Autodesk Inventor part; units mm, degrees
ref_plane "YZ Plane" through (0, 0, 0) normal (1, 0, 0) x (0, 1, 0)
ref_plane "XZ Plane" through (0, 0, 0) normal (0, 1, 0) x (-1, 0, 0)
ref_plane "XY Plane" through (0, 0, 0) normal (0, 0, 1) x (1, 0, 0)
sketch "Sketch1" plane through (0, 0, 0) normal (0, 0, 1) x (1, 0, 0)
  circle A0 centre (0, 0) radius 17.5
  dimension "d0" = 35
extrude "Extrusion1" add sketch "Sketch1" along normal blind 6
sketch "Sketch7" plane through (0, 0, 6) normal (0, 0, 1) x (1, 0, 0)
  circle A0 centre (0, 0) radius 17.5 construction
  line L0 (0, 0) -> (15, 0) construction
  circle A1 centre (0, 0) radius 17.5
  arc A2 (21.3853, 0.9) -> (17.3853, 2) centre (15.4462, -12.8741) ccw
  arc A3 (21.3853, -0.9) -> (21.3853, 0.9) centre (1.4056, 0) ccw
  arc A4 (17.3853, -2) -> (21.3853, -0.9) centre (15.4462, 12.8741) ccw
  arc A5 (17.3853, -2) -> (17.3853, 2) centre (0, 0) ccw
  arc A6 (20.2655, 6.8885) -> (16.1176, 6.817) centre (18.4476, -8.0009) ccw
  arc A7 (17.2446, 2.979) -> (16.1176, 6.817) centre (0, 0) ccw
  arc A8 (17.2446, 2.979) -> (20.7726, 5.1614) centre (11.1935, 16.7043) ccw
  arc A9 (20.7726, 5.1614) -> (20.2655, 6.8885) centre (1.3487, 0.396) ccw
  arc A10 (17.5039, 12.3189) -> (13.5442, 11.0817) centre (19.9545, -2.4796) ccw
  arc A11 (15.7068, 7.7167) -> (13.5442, 11.0817) centre (0, 0) ccw
  arc A12 (15.7068, 7.7167) -> (18.4771, 10.8047) centre (6.0339, 19.1813) ccw
  arc A13 (18.4771, 10.8047) -> (17.5039, 12.3189) centre (1.1825, 0.7599) ccw
  arc A14 (13.3242, 16.7513) -> (9.8735, 14.4487) centre (19.8447, 3.2427) ccw
  arc A15 (12.8965, 11.8292) -> (9.8735, 14.4487) centre (0, 0) ccw
  arc A16 (12.8965, 11.8292) -> (14.6846, 15.5726) centre (0.3855, 20.1042) ccw
  arc A17 (14.6846, 15.5726) -> (13.3242, 16.7513) centre (0.9205, 1.0623) ccw
  arc A18 (8.0651, 19.8267) -> (5.4029, 16.6451) centre (18.1273, 8.7023) ccw
  arc A19 (9.0414, 14.9834) -> (5.4029, 16.6451) centre (0, 0) ccw
  arc A20 (9.0414, 14.9834) -> (9.7025, 19.0789) centre (-5.2941, 19.3985) ccw
  arc A21 (9.7025, 19.0789) -> (8.0651, 19.8267) centre (0.5839, 1.2786) ccw
  arc A22 (2.1526, 21.2958) -> (0.4945, 17.493) centre (14.9413, 13.4568) ccw
  arc A23 (4.4538, 16.9238) -> (0.4945, 17.493) centre (0, 0) ccw
  arc A24 (4.4538, 16.9238) -> (3.9343, 21.0396) centre (-10.5449, 17.1212) ccw
  arc A25 (3.9343, 21.0396) -> (2.1526, 21.2958) centre (0.2, 1.3913) ccw
  arc A26 (-3.9343, 21.0396) -> (-4.4538, 16.9238) centre (10.5449, 17.1212) ccw
  arc A27 (-0.4945, 17.493) -> (-4.4538, 16.9238) centre (0, 0) ccw
  arc A28 (-0.4945, 17.493) -> (-2.1526, 21.2958) centre (-14.9413, 13.4568) ccw
  arc A29 (-2.1526, 21.2958) -> (-3.9343, 21.0396) centre (-0.2, 1.3913) ccw
  arc A30 (-9.7025, 19.0789) -> (-9.0414, 14.9834) centre (5.2941, 19.3985) ccw
  arc A31 (-5.4029, 16.6451) -> (-9.0414, 14.9834) centre (0, 0) ccw
  arc A32 (-5.4029, 16.6451) -> (-8.0651, 19.8267) centre (-18.1273, 8.7023) ccw
  arc A33 (-8.0651, 19.8267) -> (-9.7025, 19.0789) centre (-0.5839, 1.2786) ccw
  arc A34 (-14.6846, 15.5726) -> (-12.8965, 11.8292) centre (-0.3855, 20.1042) ccw
  arc A35 (-9.8735, 14.4487) -> (-12.8965, 11.8292) centre (0, 0) ccw
  arc A36 (-9.8735, 14.4487) -> (-13.3242, 16.7513) centre (-19.8447, 3.2427) ccw
  arc A37 (-13.3242, 16.7513) -> (-14.6846, 15.5726) centre (-0.9205, 1.0623) ccw
  arc A38 (-18.4771, 10.8047) -> (-15.7068, 7.7167) centre (-6.0339, 19.1813) ccw
  arc A39 (-13.5442, 11.0817) -> (-15.7068, 7.7167) centre (0, 0) ccw
  arc A40 (-13.5442, 11.0817) -> (-17.5039, 12.3189) centre (-19.9545, -2.4796) ccw
  arc A41 (-17.5039, 12.3189) -> (-18.4771, 10.8047) centre (-1.1825, 0.7599) ccw
  arc A42 (-20.7726, 5.1614) -> (-17.2446, 2.979) centre (-11.1935, 16.7043) ccw
  arc A43 (-16.1176, 6.817) -> (-17.2446, 2.979) centre (0, 0) ccw
  arc A44 (-16.1176, 6.817) -> (-20.2655, 6.8885) centre (-18.4476, -8.0009) ccw
  arc A45 (-20.2655, 6.8885) -> (-20.7726, 5.1614) centre (-1.3487, 0.396) ccw
  arc A46 (-21.3853, -0.9) -> (-17.3853, -2) centre (-15.4462, 12.8741) ccw
  arc A47 (-17.3853, 2) -> (-17.3853, -2) centre (0, 0) ccw
  arc A48 (-17.3853, 2) -> (-21.3853, 0.9) centre (-15.4462, -12.8741) ccw
  arc A49 (-21.3853, 0.9) -> (-21.3853, -0.9) centre (-1.4056, 0) ccw
  arc A50 (-20.2655, -6.8885) -> (-16.1176, -6.817) centre (-18.4476, 8.0009) ccw
  arc A51 (-17.2446, -2.979) -> (-16.1176, -6.817) centre (0, 0) ccw
  arc A52 (-17.2446, -2.979) -> (-20.7726, -5.1614) centre (-11.1935, -16.7043) ccw
  arc A53 (-20.7726, -5.1614) -> (-20.2655, -6.8885) centre (-1.3487, -0.396) ccw
  arc A54 (-17.5039, -12.3189) -> (-13.5442, -11.0817) centre (-19.9545, 2.4796) ccw
  arc A55 (-15.7068, -7.7167) -> (-13.5442, -11.0817) centre (0, 0) ccw
  arc A56 (-15.7068, -7.7167) -> (-18.4771, -10.8047) centre (-6.0339, -19.1813) ccw
  arc A57 (-18.4771, -10.8047) -> (-17.5039, -12.3189) centre (-1.1825, -0.7599) ccw
  arc A58 (-13.3242, -16.7513) -> (-9.8735, -14.4487) centre (-19.8447, -3.2427) ccw
  arc A59 (-12.8965, -11.8292) -> (-9.8735, -14.4487) centre (0, 0) ccw
  arc A60 (-12.8965, -11.8292) -> (-14.6846, -15.5726) centre (-0.3855, -20.1042) ccw
  arc A61 (-14.6846, -15.5726) -> (-13.3242, -16.7513) centre (-0.9205, -1.0623) ccw
  arc A62 (-8.0651, -19.8267) -> (-5.4029, -16.6451) centre (-18.1273, -8.7023) ccw
  arc A63 (-9.0414, -14.9834) -> (-5.4029, -16.6451) centre (0, 0) ccw
  arc A64 (-9.0414, -14.9834) -> (-9.7025, -19.0789) centre (5.2941, -19.3985) ccw
  arc A65 (-9.7025, -19.0789) -> (-8.0651, -19.8267) centre (-0.5839, -1.2786) ccw
  arc A66 (-2.1526, -21.2958) -> (-0.4945, -17.493) centre (-14.9413, -13.4568) ccw
  arc A67 (-4.4538, -16.9238) -> (-0.4945, -17.493) centre (0, 0) ccw
  arc A68 (-4.4538, -16.9238) -> (-3.9343, -21.0396) centre (10.5449, -17.1212) ccw
  arc A69 (-3.9343, -21.0396) -> (-2.1526, -21.2958) centre (-0.2, -1.3913) ccw
  arc A70 (3.9343, -21.0396) -> (4.4538, -16.9238) centre (-10.5449, -17.1212) ccw
  arc A71 (0.4945, -17.493) -> (4.4538, -16.9238) centre (0, 0) ccw
  arc A72 (0.4945, -17.493) -> (2.1526, -21.2958) centre (14.9413, -13.4568) ccw
  arc A73 (2.1526, -21.2958) -> (3.9343, -21.0396) centre (0.2, -1.3913) ccw
  arc A74 (9.7025, -19.0789) -> (9.0414, -14.9834) centre (-5.2941, -19.3985) ccw
  arc A75 (5.4029, -16.6451) -> (9.0414, -14.9834) centre (0, 0) ccw
  arc A76 (5.4029, -16.6451) -> (8.0651, -19.8267) centre (18.1273, -8.7023) ccw
  arc A77 (8.0651, -19.8267) -> (9.7025, -19.0789) centre (0.5839, -1.2786) ccw
  arc A78 (14.6846, -15.5726) -> (12.8965, -11.8292) centre (0.3855, -20.1042) ccw
  arc A79 (9.8735, -14.4487) -> (12.8965, -11.8292) centre (0, 0) ccw
  arc A80 (9.8735, -14.4487) -> (13.3242, -16.7513) centre (19.8447, -3.2427) ccw
  arc A81 (13.3242, -16.7513) -> (14.6846, -15.5726) centre (0.9205, -1.0623) ccw
  arc A82 (18.4771, -10.8047) -> (15.7068, -7.7167) centre (6.0339, -19.1813) ccw
  arc A83 (13.5442, -11.0817) -> (15.7068, -7.7167) centre (0, 0) ccw
  arc A84 (13.5442, -11.0817) -> (17.5039, -12.3189) centre (19.9545, 2.4796) ccw
  arc A85 (17.5039, -12.3189) -> (18.4771, -10.8047) centre (1.1825, -0.7599) ccw
  arc A86 (20.7726, -5.1614) -> (17.2446, -2.979) centre (11.1935, -16.7043) ccw
  arc A87 (16.1176, -6.817) -> (17.2446, -2.979) centre (0, 0) ccw
  arc A88 (16.1176, -6.817) -> (20.2655, -6.8885) centre (18.4476, 8.0009) ccw
  arc A89 (20.2655, -6.8885) -> (20.7726, -5.1614) centre (1.3487, -0.396) ccw
  point P0 (21.4056, 0)
  point P1 (20.5385, 6.0307)
  point P2 (18.0075, 11.5727)
  point P3 (14.0177, 16.1773)
  point P4 (8.8922, 19.4712)
  point P5 (3.0463, 21.1877)
  point P6 (-3.0463, 21.1877)
  point P7 (-8.8922, 19.4712)
  point P8 (-14.0177, 16.1773)
  point P9 (-18.0075, 11.5727)
  point P10 (-20.5385, 6.0307)
  point P11 (-21.4056, 0)
  point P12 (-20.5385, -6.0307)
  point P13 (-18.0075, -11.5727)
  point P14 (-14.0177, -16.1773)
  point P15 (-8.8922, -19.4712)
  point P16 (-3.0463, -21.1877)
  point P17 (3.0463, -21.1877)
  point P18 (8.8922, -19.4712)
  point P19 (14.0177, -16.1773)
  point P20 (18.0075, -11.5727)
  point P21 (20.5385, -6.0307)
  dimension "d19" = 15
  dimension "d20" = 15
  dimension "d21" = 20
  dimension "d22" = 1.8
  dimension "d23" = 2
  dimension "d24" = 4
  dimension "d27" = 360
extrude "Extrusion7" add sketch "Sketch7" against normal blind 6 contours A1 A2 A3 A4 | A1 A6 A9 A8 | A86 A89 A88 A1 | A1 A10 A13 A12 | A82 A85 A84 A1 | A1 A14 A17 A16 | A78 A81 A80 A1 | A1 A18 A21 A20 | A74 A77 A76 A1 | A1 A22 A25 A24 | A70 A73 A72 A1 | A1 A26 A29 A28 | A66 A69 A68 A1 | A1 A30 A33 A32 | A62 A65 A64 A1 | A1 A34 A37 A36 | A58 A61 A60 A1 | A1 A38 A41 A40 | A54 A57 A56 A1 | A1 A42 A45 A44 | A50 A53 A52 A1 | A1 A46 A49 A48
sketch "Sketch9" plane through (0, 0, 6) normal (0, 0, 1) x (1, 0, 0)
  circle A0 centre (0, 0) radius 11
  dimension "d33" = 22
extrude "Extrusion9" cut sketch "Sketch9" against normal through all
properties part number "Motor Coupler" material "ABS Plastic"
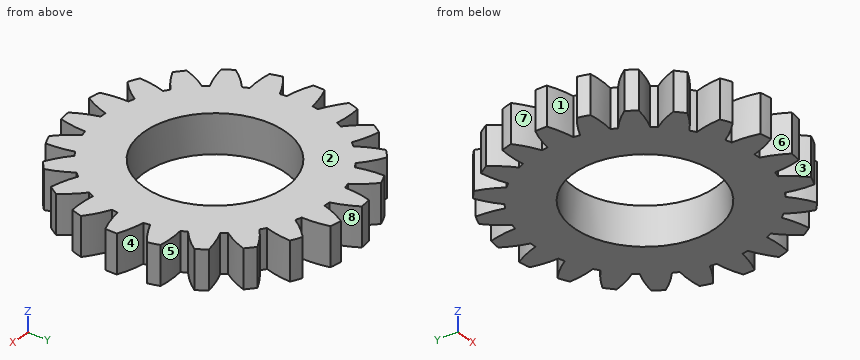
Can you work these out from the model? Positions are in its coordinate system, mm. Face numbers are marked on the shaded views. A direction names the side the tool comes from. Coordinates: 2 decimals unless noted, no trailing zeros. Write each loop counter-clockwise with the first axis right and the second up, starting at its lowest first coordinate (ties: lowest second). Pieces come first, ordered by that corner, then holes.
Q1. Imagine slicing it at B-B, the plane x = 0. List the corners of the cut face in (y, z) for me.
Results found:
outline: (-17.5, 0) - (-11, 0) - (-11, 6) - (-17.5, 6) - close; (11, 0) - (17.5, 0) - (17.5, 6) - (11, 6) - close
Q2. Please list where these lines run through material, in increasing order: L1, parallel to Y at x = 0, z = 1.45; L2, parallel to X at y = -16, z = 3.4; L3, parallel to Y at x = 19, z = 2.2.
Results found:
L1: y = -17.5 to -11, 11 to 17.5
L2: x = -14.22 to -11.95, -9.32 to 9.32, 11.95 to 14.22
L3: y = -6.99 to -3.9, -1.7 to 1.7, 3.9 to 6.99
Q3. If we mould it in two halves opening along Y, with no side actions, what happens to the marked faces 1, 2 and 3? For each: +Y half, -Y half, draft (parallel to the pull), parting line (faces both ways), or undercut.
Results found:
face 1: undercut
face 2: draft
face 3: -Y half
Q4. Imagine slicing it at A-A, the plane y = 0. List the corners of the cut face in (x, z) for me, plus the area to 3 significant figures.
Results found:
outline: (-21.41, 0) - (-11, 0) - (-11, 6) - (-21.41, 6) - close; (11, 0) - (21.41, 0) - (21.41, 6) - (11, 6) - close
area: 125 mm2
Q5. Imagine slicing it at C-C, the plane y = -18.5. List the corners of the cut face in (x, z) for me.
Results found:
outline: (-9.68, 0) - (-6.77, 0) - (-6.77, 6) - (-9.68, 6) - close; (-4.39, 0) - (-0.81, 0) - (-0.81, 6) - (-4.39, 6) - close; (0.81, 0) - (4.39, 0) - (4.39, 6) - (0.81, 6) - close; (6.77, 0) - (9.68, 0) - (9.68, 6) - (6.77, 6) - close
Q6. For P1, Ø1.5, axis at x = -14.5, z = 5.5, coming from the +Y side; P2, Ø3, axis at x = -11, z = 3.5, coming from the +Y side; P3, Ø2, axis at x = -7.5, z = 1, coming from the +Y side, each with a flat end and sliding along its axis, tell me the tip position at first contact or that it passes through.
Results found:
P1: stops at y = 16.41
P2: stops at y = 19.18
P3: stops at y = 19.83
Q7. Which directions (+Z, -Z, +X, -X, +Y, -Y) give clear straight access to the entire face, cutting with the end or side of a thin tool? Please do the marked faces 4, 5, 6, 7 and 8.
Results found:
face 4: +Z, -Z, +X
face 5: +Z, -Z
face 6: +Z, -Z, -Y
face 7: +Z, -Z, -X
face 8: +Z, -Z, +Y
